Here's how the part is built. I have some questions about the finished solid (model axes, mm). Face numbers are marked on the shaded views. Coordinates: 2 decimals unless noted, no trailing zeros. Order: outer loops, then holes, each group sorted by start corner. A loop starts at its lowest first (then second) coordinate and runs counter-clockwise, first axis right, second up. Notation, with made-up numbers: (64, 10) - (109, 10) arc R27 ccw to (109, 28) - close; hole circle Ø10 at (63.5, -30.75). An arc over 180 degrees is marked (long way). Answer as CSV lines item,"result". Start each with the question number.
Item 1: Imagine slicing it at A-A on z = -12.7. List the corners of the cut face in (x, y) for me (3 decimals), and give its area (3 significant figures).
Item 2: I'm going to push a flat-ended pin straight in: pin 1 (2.5 mm diameter, centred on x = 9.525, y = -6.35, fed in from -Z). Where does the tip first touch, or does it pass through?
Item 3: We'd pull the mould along Y, two halves only. Please class the marked faces 1, 2, 3 and 4: pulls with the +Y half, pulls with the -Y half, needs draft (parallel to the pull), parting line crosses it, or undercut.
Item 4: I need wall thicknesses on line 1 (Y direction, x = 13, z = -12.7) (3 decimals); line 2 (Y direction, x = 10, z = -14.75) (3 decimals); line 3 (Y direction, x = 15.5, z = -14.25) (3 decimals). Which ranges of each line are inside material? Lowest first, please.
Item 5: Imagine slicing it at D-D on z = -9. List the corners of the cut face in (x, y) for me (3 decimals).
Item 6: Imagine slicing it at C-C on x = 1. List the corners of the cut face in (y, z) for me (3 decimals).
Item 7: Imagine slicing it at B-B on y = -12.7. List the corners of the cut face in (x, z) for me, and give its area (3 significant figures).
from build123d import *

# Parameters (mm, degrees)
SKETCH1_W              = 19.05
SKETCH1_H              = 19.05
BOSS_EXTRUDE1_DEPTH    = 22.225
SKETCH2_R              = 2.5527
CUT_EXTRUDE1_DEPTH     = 35.925
F_10_32_TAPPED_HOLE1_D = 4.0386


with BuildPart() as part:
    # Sketch1 → Boss-Extrude1 (new, symmetric)
    with BuildSketch(Plane(origin=(0, 0, 0), x_dir=(1, 0, 0), z_dir=(0, 1, 0))):
        with Locations((9.525, 9.525)):
            Rectangle(SKETCH1_W, SKETCH1_H)
    extrude(amount=BOSS_EXTRUDE1_DEPTH, both=True)

    # Sketch2 → Cut-Extrude1 (cut, through all)
    with BuildSketch(Plane.ZY):
        with Locations((-12.7, 12.7)):
            Circle(SKETCH2_R)
        with Locations((-12.7, -12.7)):
            Circle(SKETCH2_R)
        with Locations((-12.7, 0)):
            Circle(SKETCH2_R)
    extrude(amount=-CUT_EXTRUDE1_DEPTH, mode=Mode.SUBTRACT)

    # #10-32 Tapped Hole1 (through all)
    with Locations(Plane(origin=(9.525, -6.35, -19.05), x_dir=(-1, 0, 0), z_dir=(0, 0, -1))):
        with Locations((0, 0), (0, 12.7)):
            Hole(F_10_32_TAPPED_HOLE1_D / 2)


solid = part.part
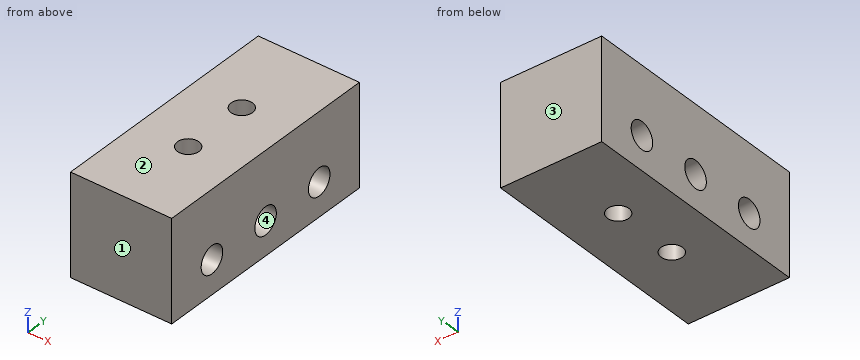
Responses:
1,outline,"(0, -22.225) - (19.05, -22.225) - (19.05, -15.253) - (0, -15.253) - close; (0, -10.147) - (19.05, -10.147) - (19.05, -2.553) - (0, -2.553) - close; (0, 2.553) - (19.05, 2.553) - (19.05, 10.147) - (0, 10.147) - close; (0, 15.253) - (19.05, 15.253) - (19.05, 22.225) - (0, 22.225) - close; hole circle Ø4.039 at (9.525, -6.35); hole circle Ø4.039 at (9.525, 6.35)"
1,area,"529 mm^2"
2,pin 1,"passes through"
3,face 1,"pulls with the -Y half"
3,face 2,"needs draft"
3,face 3,"pulls with the +Y half"
3,face 4,"undercut"
4,line 1,"y = -22.225 to -15.253, -10.147 to -2.553, 2.553 to 10.147, 15.253 to 22.225"
4,line 2,"y = -22.225 to -14.221, -11.179 to -8.313, -4.387 to -1.521, 1.521 to 4.387, 8.313 to 11.179, 14.221 to 22.225"
4,line 3,"y = -22.225 to -14.728, -10.672 to -2.028, 2.028 to 10.672, 14.728 to 22.225"
5,outline,"(0, -22.225) - (19.05, -22.225) - (19.05, 22.225) - (0, 22.225) - close; hole circle Ø4.039 at (9.525, -6.35); hole circle Ø4.039 at (9.525, 6.35)"
6,outline,"(-22.225, -19.05) - (22.225, -19.05) - (22.225, 0) - (-22.225, 0) - close; hole circle Ø5.105 at (-12.7, -12.7); hole circle Ø5.105 at (0, -12.7); hole circle Ø5.105 at (12.7, -12.7)"
7,outline,"(0, -19.05) - (19.05, -19.05) - (19.05, -15.25) - (0, -15.25) - close; (0, -10.15) - (19.05, -10.15) - (19.05, 0) - (0, 0) - close"
7,area,"266 mm^2"
